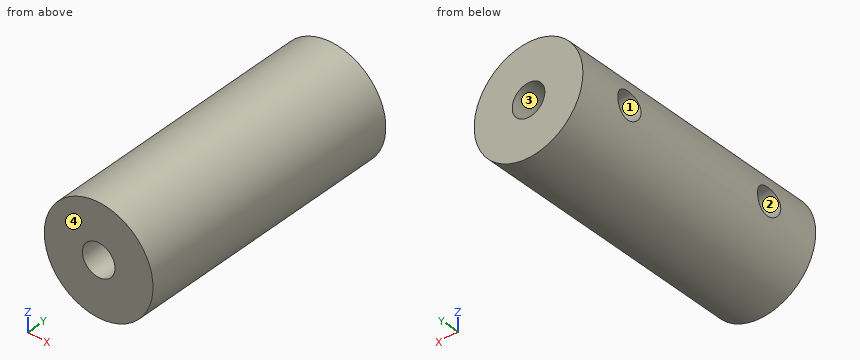
Autodesk Inventor part; units mm, degrees
ref_plane "YZ Plane" through (0, 0, 0) normal (1, 0, 0) x (0, 1, 0)
ref_plane "XZ Plane" through (0, 0, 0) normal (0, 1, 0) x (-1, 0, 0)
ref_plane "XY Plane" through (0, 0, 0) normal (0, 0, 1) x (1, 0, 0)
sketch "Sketch1" plane through (0, 0, 0) normal (0, 1, 0) x (-1, 0, 0)
  circle A0 centre (0, 0) radius 0.6
  circle A1 centre (0, 0) radius 2
  dimension "d0" = 4
  dimension "d1" = 1.2
extrude "Extrusion1" add sketch "Sketch1" along normal mid plane 10
sketch "Sketch2" plane through (0, 0, 0) normal (1, 0, 0) x (0, 1, 0)
  circle A0 centre (3, 0) radius 0.5
  point P0 (0, 0)
  dimension "d4" = 3
  dimension "d5" = 1
extrude "Extrusion2" cut sketch "Sketch2" against normal through all
mirror "Mirror1" about plane through (0, 0, 0) normal (0, 1, 0) of "Extrusion2"
properties part number "wire_connector" material "Stainless Steel"
Could you check a few things on this model? Use its own coordinates, in mm. Face numbers are marked on the shaded views. Give positions to 0.01 mm unless a question says otherwise; leave off trailing zeros. Write each loop counter-clockwise with the first axis right and the second up, starting at its lowest first coordinate (ties: lowest second). Pieces come first, ordered by that corner, then holes. Notation, with made-up numbers: (11, 44) -> (29, 44) arc R19 ccw to (29, 65) -> close; hole circle Ø10 at (-2, 13.5). An arc over 180 degrees is marked (long way). Answer as a JSON object with one key per item and string values.
Q1. Suppose I cut it at A-A on z = 0. Write out the boundary of the cut face in (x, y).
Taken from the geometry:
{"outline": "(-2, -5) -> (-0.6, -5) -> (-0.6, -3.5) -> (-2, -3.5) -> close; (-2, -2.5) -> (-0.6, -2.5) -> (-0.6, 2.5) -> (-2, 2.5) -> close; (-2, 3.5) -> (-0.6, 3.5) -> (-0.6, 5) -> (-2, 5) -> close; (0.6, -5) -> (2, -5) -> (2, 5) -> (0.6, 5) -> close"}
Q2. Suppose I cut it at B-B on x = 0. Write out the boundary of the cut face in (y, z).
Taken from the geometry:
{"outline": "(-5, -2) -> (5, -2) -> (5, -0.6) -> (-5, -0.6) -> close; (-5, 0.6) -> (5, 0.6) -> (5, 2) -> (-5, 2) -> close"}
Q3. Please list where these lines run through material, in increasing order: L1, parallel to Y at x = -1.55, z = 0; L2, parallel to Z at x = 0, y = -3; L3, parallel to Z at x = -1.15, y = -3.
Taken from the geometry:
{"L1": "y = -5 to -3.5, -2.5 to 2.5, 3.5 to 5", "L2": "z = -2 to -0.6, 0.6 to 2", "L3": "z = -1.64 to -0.5, 0.5 to 1.64"}
Q4. Will these pins go through, and if not, where does the flat tip stop? pin 1 Ø1 at (y, z) = (-2.5, -1) entering from -X; pin 2 Ø1.5 at (x, y) = (1.5, -3) entering from +Z.
Taken from the geometry:
{"pin 1": "stops at x = -1.94", "pin 2": "stops at z = 1.85"}
Q5. Suppose I cut it at D-D on z = -1.2. Write out the boundary of the cut face in (x, y), then the cut area to 3 significant figures.
Taken from the geometry:
{"outline": "(-1.6, -5) -> (1.6, -5) -> (1.6, 5) -> (-1.6, 5) -> close", "area": "32.0 mm²"}
Q6. We'd pull the mould along Y, two halves only. Please class the marked faces 1, 2, 3 and 4: released by +Y, released by -Y, zero draft, split by the parting line, or undercut.
Taken from the geometry:
{"face 1": "undercut", "face 2": "undercut", "face 3": "zero draft", "face 4": "released by -Y"}
Q7. Suppose I cut it at C-C on y = -1.5. Write out the boundary of the cut face in (x, z).
Taken from the geometry:
{"outline": "circle Ø4 at (0, 0); hole circle Ø1.2 at (0, 0)"}
